```python
from build123d import *

# Parameters (mm, degrees)
SKETCH1_W                            = 90
SKETCH1_H                            = 50
BOSS_EXTRUDE1_DEPTH                  = 5
F_5_5_5_5_DIAMETER_SLOT1_DEPTH       = 5
F_3_5_3_5_DIAMETER_HOLE1_D           = 3.5
F_3_5_3_5_DIAMETER_HOLE1_CSINK_D     = 3.55
F_3_5_3_5_DIAMETER_HOLE1_CSINK_ANGLE = 90


with BuildPart() as part:
    # Sketch1 → Boss-Extrude1 (new body)
    with BuildSketch(Plane.XY):
        Rectangle(SKETCH1_W, SKETCH1_H)
    extrude(amount=BOSS_EXTRUDE1_DEPTH)

    # Ø5.5 (5.5) Diameter Slot1: read off the stored shape, not the designer's step
    # Ø5.5 (5.5) Diameter Slot1 outline → Ø5.5 (5.5) Diameter Slot1 (cut)
    with BuildSketch(Plane.XY):
        with BuildLine():
            ThreePointArc((32.25, -2.75), (35, 0), (32.25, 2.75))
            Line((32.25, 2.75), (-32.25, 2.75))
            ThreePointArc((-32.25, 2.75), (-35, 0), (-32.25, -2.75))
            Line((-32.25, -2.75), (32.25, -2.75))
        make_face()
    extrude(amount=F_5_5_5_5_DIAMETER_SLOT1_DEPTH, mode=Mode.SUBTRACT)

    # 5.5 _5.5_ Diameter Slot1 2: loft between two sections, ruled curve by curve
    f_5_5_5_5_diameter_slot1_2_from = [
        Edge.make_three_point_arc((32.25, 2.75, 0.025), (34.194543648, 1.944543648, 0.025), (35, 0, 0.025)),
        Edge.make_three_point_arc((35, 0, 0.025), (34.194543648, -1.944543648, 0.025), (32.25, -2.75, 0.025)),
        Edge.make_three_point_arc((-32.25, -2.75, 0.025), (-34.194543648, -1.944543648, 0.025), (-35, 0, 0.025)),
        Edge.make_three_point_arc((-35, 0, 0.025), (-34.194543648, 1.944543648, 0.025), (-32.25, 2.75, 0.025)),
        Edge.make_line((32.25, -2.75, 0.025), (-32.25, -2.75, 0.025)),
        Edge.make_line((32.25, 2.75, 0.025), (-32.25, 2.75, 0.025)),
    ]
    f_5_5_5_5_diameter_slot1_2_to = [
        Edge.make_three_point_arc((32.25, 2.775, 0), (34.212221318, 1.962221318, 0), (35.025, 0, 0)),
        Edge.make_three_point_arc((35.025, 0, 0), (34.212221318, -1.962221318, 0), (32.25, -2.775, 0)),
        Edge.make_three_point_arc((-32.25, -2.775, 0), (-34.212221318, -1.962221318, 0), (-35.025, 0, 0)),
        Edge.make_three_point_arc((-35.025, 0, 0), (-34.212221318, 1.962221318, 0), (-32.25, 2.775, 0)),
        Edge.make_line((32.25, -2.775, 0), (-32.25, -2.775, 0)),
        Edge.make_line((32.25, 2.775, 0), (-32.25, 2.775, 0)),
    ]
    f_5_5_5_5_diameter_slot1_2 = Solid(Shell([*[Face.make_surface_from_curves(f_5_5_5_5_diameter_slot1_2_from[k], f_5_5_5_5_diameter_slot1_2_to[k]) for k in range(6)], Face(Wire(f_5_5_5_5_diameter_slot1_2_from)), Face(Wire(f_5_5_5_5_diameter_slot1_2_to))]))
    add(f_5_5_5_5_diameter_slot1_2, mode=Mode.SUBTRACT)

    # Ø3.5 (3.5) Diameter Hole1 (through all)
    with Locations(Plane(origin=(0, 0, 0), x_dir=(-1, 0, 0), z_dir=(0, 0, -1))):
        with Locations((-40, 20), (40, 20), (40, -20), (-40, -20)):
            CounterSinkHole(F_3_5_3_5_DIAMETER_HOLE1_D / 2, F_3_5_3_5_DIAMETER_HOLE1_CSINK_D / 2, counter_sink_angle=F_3_5_3_5_DIAMETER_HOLE1_CSINK_ANGLE)


solid = part.part
```
Can you work these out from the model? Positions are in its coordinate system, mm. A direction names the side the tool comes from. Round coordinates to 2 decimals unless told otherwise and drop trailing zeros. Loops run counter-clockwise (first coordinate to the right, second up) from the corner with the lowest first, then second, coordinate; pieces in that order, holes last. Notation, with made-up numbers: M -33,-18.5 L 20,-18.5 A22 cw 20,5.5 Z; hole C 42.5,37 d4. An arc over 180 degrees is marked long. Answer as a JSON object with one key per item and string values. Group by question number.
Q1. Imagine slicing it at A-A, the plane x = 40. Please give me the cut outline in (y, z) (3 decimals).
Q2. Will this pin go through, and if not, where does the flat tip stop? pin 1 (3 mm diameter, centred on x = 40, y = 20, fed in from +Z).
Q3. Imagine slicing it at B-B, the plane z = 0.8. Please give me the cut outline in (x, y).
Q4. Please list where these lines run through material, in increasing order: L1, parallel to Y at x = -40, z = 1; L2, parallel to X at y = 20, z = 1.55; L3, parallel to Y at x = -21, z = 4.75.
Q5. On a 3-axis mill with a long thin cutter (end or side, diameter ignored), from which of +Z, -Z, +X, -X, +Y, -Y can I reach the whole of each face in a straight line? I mean faces 1 (the flat face through (0, 2.75, 2)), 2 (the flat face through (-45, 0, 2)). Say none if no direction works.
Q6. We'd pull the mould along Y, two halves only. Please class faces 3 (the cylindrical face through (-39.1, -18.5, 2.5)), 4 (the flat face through (-1, -25, 2)), 5 (the flat face through (45, 0, 2)), 6 (the flat face through (-1, 25, 2)): +Y half, -Y half, draft (parallel to the pull), parting line (faces both ways), or undercut.
Findings:
{
 "1": {"outline": "M -25,0 L -21.775,0 L -21.75,0.025 L -21.75,5 L -25,5 Z; M -18.25,0.025 L -18.225,0 L 18.225,0 L 18.25,0.025 L 18.25,5 L -18.25,5 Z; M 21.75,0.025 L 21.775,0 L 25,0 L 25,5 L 21.75,5 Z"},
 "2": {"pin 1": "passes through"},
 "3": {"outline": "M -45,-25 L 45,-25 L 45,25 L -45,25 Z; hole C -40,-20 d3.5; hole C -40,20 d3.5; hole M -32.25,-2.75 L 32.25,-2.75 A2.75 ccw 32.25,2.75 L -32.25,2.75 A2.75 ccw Z; hole C 40,-20 d3.5; hole C 40,20 d3.5"},
 "4": {"L1": "y = -25 to -21.75, -18.25 to 18.25, 21.75 to 25", "L2": "x = -45 to -41.75, -38.25 to 38.25, 41.75 to 45", "L3": "y = -25 to -2.75, 2.75 to 25"},
 "5": {"face 1": "+Z, -Z", "face 2": "+Z, -Z, -X, +Y, -Y"},
 "6": {"face 3": "undercut", "face 4": "-Y half", "face 5": "draft", "face 6": "+Y half"}
}
